```python
from build123d import *

# Parameters (mm, degrees)
F0_W     = 150
F0_H     = 150
F1_DEPTH = 17.5
F3_DEPTH = 150.001
F5_DEPTH = 150.001
F6_R     = 5


with BuildPart() as f1:
    # F0 (on Top) → F1 (new body, symmetric)
    with BuildSketch(Plane.XY):
        Rectangle(F0_W, F0_H)
    extrude(amount=F1_DEPTH, both=True)

    # F2 (on face) → F3 (cut, through all)
    with BuildSketch(Plane.XZ.offset(75)):
        Polygon((-8.13676, 17.5), (-12.5, 0), (12.5, 0), (8.13676, 17.5), align=None)
    extrude(amount=-F3_DEPTH, mode=Mode.SUBTRACT)

    # F4 (on face) → F5 (cut, through all)
    with BuildSketch(Plane.YZ.offset(75)):
        Polygon((-8.13676, 17.5), (-12.5, 0), (12.5, 0), (8.13676, 17.5), align=None)
    extrude(amount=-F5_DEPTH, mode=Mode.SUBTRACT)

    # F6
    f6_edges = [f1.edges().sort_by_distance(p)[0] for p in [
        (-75, 41.56838, 17.5),
        (-75, -41.56838, 17.5),
        (-41.56838, -75, 17.5),
        (41.56838, -75, 17.5),
        (75, -41.56838, 17.5),
        (75, 41.56838, 17.5),
        (41.56838, 75, 17.5),
        (-41.56838, 75, 17.5),
    ]]
    fillet(f6_edges, radius=F6_R)


solid = f1.part
```
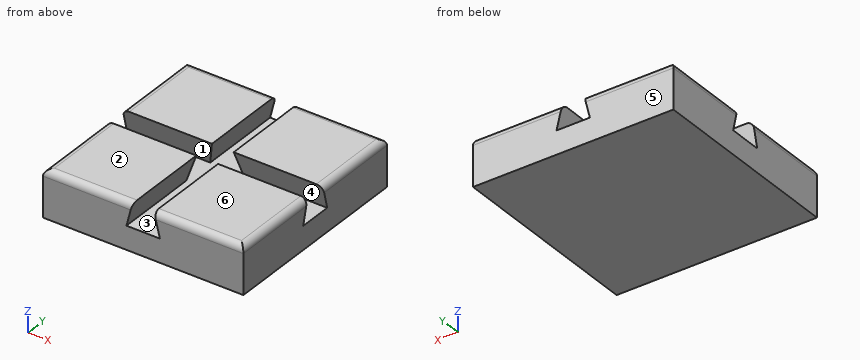
Here's how the part is built. I have some questions about the finished solid (model axes, mm). Face numbers are marked on the shaded views. A direction names the side the tool comes from. Coordinates: 2 decimals unless noted, no trailing zeros. Order: outer loops, then holes, each group sorted by start corner. A loop starts at its lowest first (then second) coordinate and runs counter-clockwise, first axis right, second up. Notation, with made-up numbers: (-34, 61) -> (22, 61) arc R22 cw to (22, 77) -> close; hole circle Ø7 at (25, -2.5). An arc over 180 degrees is marked (long way). Return JSON: item names as keys, results as strings.
1) If I drill on probe 1 along X at (y, z) = (-51, 7); probe 2 along Y at (x, z) = (30.5, 3); probe 3 along Z at (x, y) = (-4.5, -37), over which ranges is the centre line in solid material (lowest first)?
Conclusion:
{"probe 1": "x = -75 to -10.75, 10.75 to 75", "probe 2": "y = -75 to -11.75, 11.75 to 75", "probe 3": "z = -17.5 to 0"}
2) If we section it at A-A on y = 49: List the corners of the cut face in (x, z) for me.
Conclusion:
{"outline": "(-75, -17.5) -> (75, -17.5) -> (75, 12.5) arc R5 ccw to (70, 17.5) -> (8.14, 17.5) -> (12.5, 0) -> (-12.5, 0) -> (-8.14, 17.5) -> (-70, 17.5) arc R5 ccw to (-75, 12.5) -> close"}
3) Thinking about a two-plate mould opening in Z: for the marked faces 4, 5 and 6, which applies, +Z half, -Z half, draft (parallel to the pull), parting line (faces both ways), or undercut?
Conclusion:
{"face 4": "undercut", "face 5": "draft", "face 6": "+Z half"}
4) If we section it at C-C on z = 9: List the corners of the cut face in (x, y) for me, plus the area to 3 significant figures.
Conclusion:
{"outline": "(-75, -75) -> (-10.26, -75) -> (-10.26, -10.26) -> (-75, -10.26) -> close; (-75, 10.26) -> (-10.26, 10.26) -> (-10.26, 75) -> (-75, 75) -> close; (10.26, -75) -> (75, -75) -> (75, -10.26) -> (10.26, -10.26) -> close; (10.26, 10.26) -> (75, 10.26) -> (75, 75) -> (10.26, 75) -> close", "area": "16,800 mm²"}
5) On a 3-axis mill with a long thin cutter (end or side, diameter ignored), from which of +Z, -Z, +X, -X, +Y, -Y can I reach the whole of each face in a straight line? I mean the marked faces 1, 2 and 3. Say none if no direction works.
Conclusion:
{"face 1": "+X, -X", "face 2": "+Z, +X, -X, +Y, -Y", "face 3": "none"}
